The listing builds one solid part. Answer for the finished solid, in the listing's coordinates (mm). A direction names the side the tool comes from. Give positions to 0.01 mm unless a question says otherwise; leave off trailing zeros. Write each loop counter-clockwise with the first axis right and the second up, starting at its lowest first coordinate (ties: lowest second). Pieces come first, ordered by that corner, then holes. Notation, with made-up numbers: (-13.75, 52) - (-2.75, 52) arc R16 ccw to (-2.75, 56) - close; hole circle Ø8 at (41, -16.5). An arc over 180 degrees is marked (long way). One line per question, with ' | ' between items. Start each with the question number.
1. The mould has two halves that part along Z. Classify faces 3 (the face through (-69.856, -1.61, 25.121)), 4 (the face through (406.4, -1, -29)), 5 (the face through (2, 9, -63.5)): +Z half, -Z half, draft (parallel to the pull), parting line (faces both ways), or undercut.
2. A cutting plane is placed at A-A (x = -282). Determine the outline of the cut face in (y, z) (3 decimals), then the cut area to 3 significant figures.
3. For faces 1 (the face through (1.38, -1.61, 31.6)), 2 (the face through (-290, 7, -60.325)), determine the directions among +Z, -Z, +X, -X, +Y, -Y from which every point of the face is accessible in a straight line to the end or side of a thin tool.
4. Find the intervals of material crossed by L1, parallel to X at y = -1, z = -50.8; L2, parallel to Z at x = 88, y = 2.5; L3, parallel to Y at x = 89.5, z = -32 (3 decimals), in increasing order. Write a range as from..to.
5. Given P1, Ø3, axis at x = -368.3, y = 9.525, coming from the +Z side; P2, Ø1.6, axis at x = -159.5, y = -1.5, coming from the -Z side; P3, Ø10.5, axis at x = 393.7, z = 50.8, coming from the +Y side, each flat-ended and moving along its own axis, determine where each tip first touches the part or whether it passes through.
```python
from build123d import *

# Parameters (mm, degrees)
SKETCH1_W                      = 812.8
SKETCH1_H                      = 127
BASE_FLANGE1_DEPTH             = 3.175
EDGE_FLANGE1_STRIP_W           = 19.05
EDGE_FLANGE1_STRIP_H           = 3.175
EDGE_FLANGE1_STRIP_CUT_DEPTH   = 812.8
EDGE_FLANGE1_STRIP_2_W         = 19.05
EDGE_FLANGE1_STRIP_2_H         = 3.175
EDGE_FLANGE1_STRIP_CUT_2_DEPTH = 812.8
EDGE_FLANGE1_DEPTH             = 812.8
EDGE_FLANGE1_BEND_DEPTH        = 812.8
MOUNTING_HOLES_D               = 5
LPATTERN3_COUNT                = 32
LPATTERN3_PITCH                = 25.4
SKETCH21_W                     = 25.4
SKETCH21_H                     = 6.35
CUT_EXTRUDE3_DEPTH             = 412.771918057
CUT_EXTRUDE4_DEPTH             = 412.637250045
CUT_EXTRUDE4_DEPTH_BACK        = 412.637250045
F_80_20_CONNECTION_HOLES_D     = 6.6
MOTOR_HOLES_D                  = 12.7
F_1_2_0_5_DIAMETER_HOLE1_D     = 12.7
CUT_EXTRUDE5_DEPTH             = 412.637250045
F_1_0MM_DOWEL_HOLE1_D          = 6.6
F_5_0MM_DOWEL_HOLE1_D          = 5


# Sheet-metal steps are written as plain solids
with BuildPart() as part:
    # Sketch1 → Base-Flange1 (new body)
    with BuildSketch(Plane(origin=(0, 0, 0), x_dir=(1, 0, 0), z_dir=(0, 1, 0))):
        Rectangle(SKETCH1_W, SKETCH1_H)
    extrude(amount=-BASE_FLANGE1_DEPTH)

    # Edge-Flange1 strip (across the edge) → Edge-Flange1 strip cut (cut)
    with BuildSketch(Plane(origin=(406.4, 0, -63.5), x_dir=(0, 0, 1), z_dir=(-1, 0, 0))):
        with Locations((-3.175, -1.5875)):
            Rectangle(EDGE_FLANGE1_STRIP_W, EDGE_FLANGE1_STRIP_H)
    extrude(amount=EDGE_FLANGE1_STRIP_CUT_DEPTH, mode=Mode.SUBTRACT)

    # Edge-Flange1 strip 2 (across the edge) → Edge-Flange1 strip cut 2 (cut)
    with BuildSketch(Plane(origin=(-406.4, 0, 63.5), x_dir=(0, 0, -1), z_dir=(1, 0, 0))):
        with Locations((-3.175, -1.5875)):
            Rectangle(EDGE_FLANGE1_STRIP_2_W, EDGE_FLANGE1_STRIP_2_H)
    extrude(amount=EDGE_FLANGE1_STRIP_CUT_2_DEPTH, mode=Mode.SUBTRACT)

    # Edge-Flange1 section (across the edge) → Edge-Flange1 (add)
    with BuildSketch(Plane(origin=(406.4, 0, -63.5), x_dir=(0, 0, 1), z_dir=(-1, 0, 0))):
        with BuildLine():
            Line((0, 3.175), (0, 15.875))
            Line((0, 15.875), (3.175, 15.875))
            Line((3.175, 15.875), (3.175, 3.175))
            ThreePointArc((3.175, 3.175), (4.10493597, 0.92993597), (6.35, 0))
            Line((6.35, 0), (6.35, -3.175))
            ThreePointArc((6.35, -3.175), (1.859871939, -1.315128061), (0, 3.175))
        make_face()
    extrude(amount=EDGE_FLANGE1_DEPTH)

    # Edge-Flange1 section 2 (across the edge) → Edge-Flange1 bend (add)
    with BuildSketch(Plane(origin=(-406.4, 0, 63.5), x_dir=(0, 0, -1), z_dir=(1, 0, 0))):
        with BuildLine():
            Line((0, 3.175), (0, 15.875))
            Line((0, 15.875), (3.175, 15.875))
            Line((3.175, 15.875), (3.175, 3.175))
            ThreePointArc((3.175, 3.175), (4.10493597, 0.92993597), (6.35, 0))
            Line((6.35, 0), (6.35, -3.175))
            ThreePointArc((6.35, -3.175), (1.859871939, -1.315128061), (0, 3.175))
        make_face()
    extrude(amount=EDGE_FLANGE1_BEND_DEPTH)

    # Mounting Holes (through all)
    with Locations(Plane(origin=(342.9, 0, -63.5), x_dir=(1, 0, 0), z_dir=(0, 0, -1))):
        with Locations((-736.6, -9.525)):
            mounting_holes = Hole(MOUNTING_HOLES_D / 2)

    # LPattern3: Mounting Holes ×32
    with Locations(*[(i * LPATTERN3_PITCH, 0, 0) for i in range(1, LPATTERN3_COUNT)]):
        add(mounting_holes, mode=Mode.SUBTRACT)

    # Sketch21 → Cut-Extrude3 (cut, through all)
    with BuildSketch(Plane.XZ.offset(3.175)):
        with Locations((165.1, -60.325)):
            Rectangle(SKETCH21_W, SKETCH21_H)
        with Locations((-165.1, -60.325)):
            Rectangle(SKETCH21_W, SKETCH21_H)
    extrude(amount=-CUT_EXTRUDE3_DEPTH, mode=Mode.SUBTRACT)

    # Sketch26 → Cut-Extrude4 (cut, two sides: drawn at the far end of the back side and taken through both)
    with BuildSketch(Plane(origin=(0, 0, 0), x_dir=(1, 0, 0), z_dir=(0, 1, 0)).offset(-CUT_EXTRUDE4_DEPTH_BACK)):
        with BuildLine():
            Line((152.4, -57.15), (152.4, -63.5))
            Line((152.4, -63.5), (165.1, -63.5))
            Line((165.1, -63.5), (165.1, -57.15))
            ThreePointArc((165.1, -57.15), (158.75, -50.8), (152.4, -57.15))
        make_face()
        with BuildLine():
            Line((-165.1, -57.15), (-165.1, -63.5))
            Line((-165.1, -63.5), (-152.4, -63.5))
            Line((-152.4, -63.5), (-152.4, -57.15))
            ThreePointArc((-152.4, -57.15), (-158.75, -50.8), (-165.1, -57.15))
        make_face()
    extrude(amount=CUT_EXTRUDE4_DEPTH + CUT_EXTRUDE4_DEPTH_BACK, mode=Mode.SUBTRACT)

    # 80/20 Connection Holes (through all)
    with Locations(Plane(origin=(0, 0, 0), x_dir=(1, 0, 0), z_dir=(0, 1, 0))):
        with Locations((-165.1, 50.8), (165.1, 50.8), (-393.7, 0), (-393.7, -50.8), (393.7, -50.8), (393.7, 0)):
            Hole(F_80_20_CONNECTION_HOLES_D / 2)

    # Motor Holes (through all)
    with Locations(Plane(origin=(0, 0, 0), x_dir=(1, 0, 0), z_dir=(0, 1, 0))):
        with Locations((-317.5, -25.4), (317.5, -25.4)):
            Hole(MOTOR_HOLES_D / 2)

    # 1/2 (0.5) Diameter Hole1 (through all)
    with Locations(Plane(origin=(0, 0, 0), x_dir=(1, 0, 0), z_dir=(0, 1, 0))):
        with Locations((76.2, -25.4), (0, -25.4), (-25.4, -25.4), (-50.8, -25.4), (-76.2, -25.4), (25.4, -25.4), (50.8, -25.4)):
            Hole(F_1_2_0_5_DIAMETER_HOLE1_D / 2)

    # Sketch33 → Cut-Extrude5 (cut, through all)
    with BuildSketch(Plane(origin=(0, 0, 0), x_dir=(1, 0, 0), z_dir=(0, 1, 0))):
        with BuildLine():
            Line((-406.4, -19.05), (-406.4, -31.75))
            ThreePointArc((-406.4, -31.75), (-400.05, -25.4), (-406.4, -19.05))
        make_face()
        with BuildLine():
            Line((406.4, -19.05), (406.4, -31.75))
            ThreePointArc((406.4, -31.75), (400.05, -25.4), (406.4, -19.05))
        make_face()
    extrude(amount=-CUT_EXTRUDE5_DEPTH, mode=Mode.SUBTRACT)

    # Ø1.0mm Dowel Hole1 (through all)
    with Locations(Plane(origin=(0, 0, 0), x_dir=(1, 0, 0), z_dir=(0, 1, 0))):
        with Locations((88.9, -45.28), (-88.9, 45.28), (-88.9, -45.28), (88.9, 45.28)):
            Hole(F_1_0MM_DOWEL_HOLE1_D / 2)

    # Ø5.0mm Dowel Hole1 (through all)
    with Locations(Plane(origin=(0, 0, 0), x_dir=(1, 0, 0), z_dir=(0, 1, 0))):
        with Locations((172.6, 29.8), (-172.6, 29.8), (-157.6, 29.8), (157.6, 29.8)):
            Hole(F_5_0MM_DOWEL_HOLE1_D / 2)


solid = part.part
```
Determined:
1) face 3: undercut | face 4: draft | face 5: -Z half
2) outline: (-3.175, -57.15) arc R6.35 ccw to (3.175, -63.5) - (15.875, -63.5) - (15.875, -60.325) - (3.175, -60.325) arc R3.175 cw to (0, -57.15) - (0, 57.15) arc R3.175 cw to (3.175, 60.325) - (15.875, 60.325) - (15.875, 63.5) - (3.175, 63.5) arc R6.35 ccw to (-3.175, 57.15) - close | area: 491 mm2
3) face 1: +Y, -Y | face 2: +X, -X, +Y
4) L1: -406.4..-168.4, -161.8..161.8, 168.4..406.4 | L2: -63.46..-60.25, 60.25..63.46 | L3: -3.175..0
5) P1: through | P2: z = -57.15 | P3: y = 0
